The model under review builds one solid part; all positions refer to its coordinate system, in mm. A direction names the side the tool comes from. Give positions to 0.01 mm unless a question says otherwise; leave off trailing zeros. Order: outer loops, then holes, each group sorted by start corner. A loop starts at its lowest first (then second) coordinate and runs counter-clockwise, first axis right, second up. Notation, with made-up numbers: (-30, -15) - (-13, -15) arc R16 cw to (-13, 16) - close; hole circle Ø3 at (-36, 25). An arc over 180 degrees is marked (long way). Use CSV: the item, a comma, the result in double quotes.
```python
from build123d import *

# Parameters (mm, degrees)
PAD_DEPTH       = 1
PAD001_DEPTH    = 18
SKETCH002_W     = 19.2
SKETCH002_H     = 12.2
POCKET_DEPTH    = 5
SKETCH003_W     = 21.2
SKETCH003_H     = 14.2
SKETCH003_W_2   = 19.2
SKETCH003_H_2   = 12.2
PAD002_DEPTH    = 1
CHAMFER_SIZE    = 0.99
PAD003_DEPTH    = 2
CHAMFER001_SIZE = 1.8
SKETCH005_W     = 36
SKETCH005_H     = 15
PAD004_DEPTH    = 2.5
PAD004_FACE29_W = 15
PAD004_FACE29_H = 36
PAD005_DEPTH    = 10
SKETCH006_R     = 1
SKETCH006_R_2   = 0.751416
SKETCH006_R_3   = 0.769216
PAD006_DEPTH    = 1
SKETCH007_R     = 1.25
PAD007_DEPTH    = 1.2
PAD007_FACE39_W = 15
PAD007_FACE39_H = 36
POCKET001_DEPTH = 5
SKETCH008_R     = 6.15
POCKET002_DEPTH = 19
PAD008_DEPTH    = 1
PAD009_DEPTH    = 1
SKETCH009_W     = 12
SKETCH009_H     = 5
POCKET003_DEPTH = 5
FILLET_R        = 1
POCKET004_DEPTH = 5
POCKET005_DEPTH = 5


with BuildPart() as part:
    # Sketch → Pad (new body)
    with BuildSketch(Plane.XY):
        with BuildLine():
            Line((1, 0), (39, 0))
            ThreePointArc((39, 0), (39.707107, 0.292893), (40, 1))
            Line((40, 1), (40, 39))
            ThreePointArc((40, 39), (39.707107, 39.707107), (39, 40))
            Line((39, 40), (1, 40))
            ThreePointArc((1, 40), (0.292893, 39.707107), (0, 39))
            Line((0, 39), (0, 1))
            ThreePointArc((0, 1), (0.292893, 0.292893), (1, 0))
        make_face()
    extrude(amount=PAD_DEPTH)

    # Sketch001 (on Face10 of Pad) → Pad001 (join)
    with BuildSketch(Plane.XY.offset(1)):
        with BuildLine():
            Line((1, 0), (39, 0))
            ThreePointArc((39, 0), (39.707107, 0.292893), (40, 1))
            Line((40, 1), (40, 39))
            ThreePointArc((40, 39), (39.707107, 39.707107), (39, 40))
            Line((39, 40), (1, 40))
            ThreePointArc((1, 40), (0.292893, 39.707107), (0, 39))
            Line((0, 39), (0, 1))
            ThreePointArc((0, 1), (0.292893, 0.292893), (1, 0))
        make_face()
        with BuildLine():
            Line((2, 1), (38, 1))
            ThreePointArc((38, 1), (38.707107, 1.292893), (39, 2))
            Line((39, 2), (39, 38))
            ThreePointArc((39, 38), (38.707107, 38.707107), (38, 39))
            Line((38, 39), (2, 39))
            ThreePointArc((2, 39), (1.292893, 38.707107), (1, 38))
            Line((1, 38), (1, 2))
            ThreePointArc((1, 2), (1.292893, 1.292893), (2, 1))
        make_face(mode=Mode.SUBTRACT)
    extrude(amount=PAD001_DEPTH)

    # Sketch002 (on Face14 of Pad001) → Pocket (cut)
    with BuildSketch(Plane.YZ.offset(40)):
        with Locations((26.6, 11.1)):
            Rectangle(SKETCH002_W, SKETCH002_H)
    extrude(amount=-POCKET_DEPTH, mode=Mode.SUBTRACT)

    # Sketch003 (on Face17 of Pocket) → Pad002 (join)
    with BuildSketch(Plane(origin=(39, 0, 0), x_dir=(0, -1, 0), z_dir=(-1, 0, 0))):
        with Locations((-26.6, 11.1)):
            Rectangle(SKETCH003_W, SKETCH003_H)
        with Locations((-26.6, 11.1)):
            Rectangle(SKETCH003_W_2, SKETCH003_H_2, mode=Mode.SUBTRACT)
    extrude(amount=PAD002_DEPTH)

    # Chamfer
    chamfer_edges = [part.edges().sort_by_distance(p)[0] for p in [
        (38, 26.6, 18.2),
        (38, 16, 11.1),
        (38, 26.6, 4),
        (38, 37.2, 11.1),
    ]]
    chamfer(chamfer_edges, length=CHAMFER_SIZE)

    # Sketch004 (on Face11 of Chamfer) → Pad003 (join)
    with BuildSketch(Plane.XY.offset(1)):
        with BuildLine():
            Line((2, 39), (2, 18.5))
            ThreePointArc((2, 18.5), (2.292893, 17.792893), (3, 17.5))
            Line((3, 17.5), (5, 17.5))
            Line((5, 17.5), (5, 14))
            Line((5, 14), (17, 14))
            Line((17, 17.5), (17, 14))
            Line((17, 17.5), (19, 17.5))
            ThreePointArc((19, 17.5), (19.707107, 17.792893), (20, 18.5))
            Line((20, 18.5), (20, 20))
            Line((20, 20), (22, 20))
            Line((22, 20), (22, 17.5))
            Line((22, 17.5), (38, 17.5))
            Line((38, 17.5), (38, 38))
            Line((38, 38), (22, 38))
            Line((22, 38), (22, 37))
            Line((22, 37), (20, 37))
            Line((20, 37), (20, 39))
            Line((20, 39), (39, 39))
            Line((39, 1), (39, 39))
            Line((1, 1), (39, 1))
            Line((1, 39), (1, 1))
            Line((1, 39), (2, 39))
        make_face()
    extrude(amount=PAD003_DEPTH)

    # Chamfer001
    chamfer001_edges = [part.edges().sort_by_distance(p)[0] for p in [
        (11, 14, 3),
    ]]
    chamfer(chamfer001_edges, length=CHAMFER001_SIZE)

    # Sketch005 (on Face1 of Chamfer001) → Pad004 (join, symmetric)
    with BuildSketch(Plane.XY.offset(3)):
        with Locations((20, 8.5)):
            Rectangle(SKETCH005_W, SKETCH005_H)
    extrude(amount=PAD004_DEPTH, both=True)

    # Pad004 Face29 → Pad005 (add)
    with BuildSketch(Plane(origin=(20, 8.5, 5.5), x_dir=(0, 1, 0), z_dir=(0, 0, 1))):
        Rectangle(PAD004_FACE29_W, PAD004_FACE29_H)
    extrude(amount=PAD005_DEPTH)

    # Sketch006 (on Face18 of Pad005) → Pad006 (join)
    with BuildSketch(Plane.XY.offset(1)):
        with Locations((3, 18.5)):
            Circle(SKETCH006_R)
        with Locations((19, 18.5)):
            Circle(SKETCH006_R)
        with Locations((2.699211, 38.373474)):
            Circle(SKETCH006_R_2)
        with Locations((19.24682, 38.345665)):
            Circle(SKETCH006_R_3)
    extrude(amount=PAD006_DEPTH)

    # Sketch007 (on Face20 of Pad006) → Pad007 (join)
    with BuildSketch(Plane.XY.offset(1)):
        with Locations((35.5, 35.5)):
            Circle(SKETCH007_R)
        with Locations((35.5, 20)):
            Circle(SKETCH007_R)
    extrude(amount=PAD007_DEPTH)

    # Pad007 Face39 → Pocket001 (cut)
    with BuildSketch(Plane(origin=(20, 8.5, 15.5), x_dir=(0, 1, 0), z_dir=(0, 0, 1))):
        Rectangle(PAD007_FACE39_W, PAD007_FACE39_H)
    extrude(amount=-POCKET001_DEPTH, mode=Mode.SUBTRACT)

    # Sketch008 (on DatumPlane) → Pocket002 (cut, symmetric)
    with BuildSketch(Plane.YZ.offset(20)):
        with Locations((9, 11)):
            Circle(SKETCH008_R)
    extrude(amount=POCKET002_DEPTH, both=True, mode=Mode.SUBTRACT)

    # Pocket002 Face46 → Pad008 (add)
    with BuildSketch(Plane(origin=(2, 8.050341, 5.520041), x_dir=(0, 1, 0), z_dir=(-1, 0, 0))):
        with BuildLine():
            Line((7.949659, 2.520041), (-7.050341, 2.520041))
            Line((-7.050341, 2.520041), (-7.050341, -4.979959))
            Line((-7.050341, -4.979959), (-5.179982, -4.979959))
            ThreePointArc((-5.179982, -4.979959), (0.949659, 0.670041), (7.0793, -4.979959))
            Line((7.0793, -4.979959), (7.949659, -4.979959))
            Line((7.949659, -4.979959), (7.949659, 2.520041))
        make_face()
    extrude(amount=PAD008_DEPTH)

    # Pad008 Face32 → Pad009 (add)
    with BuildSketch(Plane(origin=(38, 8.050341, 5.520041), x_dir=(0, -1, 0), z_dir=(1, 0, 0))):
        with BuildLine():
            Line((7.050341, 2.520041), (-7.949659, 2.520041))
            Line((-7.949659, 2.520041), (-7.949659, -4.979959))
            Line((-7.949659, -4.979959), (-7.0793, -4.979959))
            ThreePointArc((-7.0793, -4.979959), (-0.949659, 0.670041), (5.179982, -4.979959))
            Line((5.179982, -4.979959), (7.050341, -4.979959))
            Line((7.050341, -4.979959), (7.050341, 2.520041))
        make_face()
    extrude(amount=PAD009_DEPTH)

    # Sketch009 (on Face69 of Pad009) → Pocket003 (cut)
    with BuildSketch(Plane.XY.offset(10.5)):
        with Locations((11, 13.5)):
            Rectangle(SKETCH009_W, SKETCH009_H)
    extrude(amount=-POCKET003_DEPTH, mode=Mode.SUBTRACT)

    # Fillet
    fillet_edges = [part.edges().sort_by_distance(p)[0] for p in [
        (11, 16, 5.5),
    ]]
    fillet(fillet_edges, radius=FILLET_R)

    # Sketch010 (on Face62 of Fillet) → Pocket004 (cut)
    with BuildSketch(Plane(origin=(0, 0, 0), x_dir=(0, -1, 0), z_dir=(-1, 0, 0))):
        with BuildLine():
            ThreePointArc((-22.577213, 15.673276), (-21.827213, 14.923276), (-21.077213, 15.673276))
            Line((-21.077213, 15.673276), (-21.077213, 20.673276))
            ThreePointArc((-21.077213, 20.673276), (-21.827213, 21.423276), (-22.577213, 20.673276))
            Line((-22.577213, 15.673276), (-22.577213, 20.673276))
        make_face()
    extrude(amount=-POCKET004_DEPTH, mode=Mode.SUBTRACT)

    # Sketch013 (on Face63 of Pocket004) → Pocket005 (cut)
    with BuildSketch(Plane(origin=(0, 40, 0), x_dir=(-1, 0, 0), z_dir=(0, 1, 0))):
        with BuildLine():
            Line((-6.1, 4), (-6.1, 6))
            ThreePointArc((-6.1, 6), (-6.392893, 6.707107), (-7.1, 7))
            Line((-7.1, 7), (-15.1, 7))
            ThreePointArc((-15.1, 7), (-15.807107, 6.707107), (-16.1, 6))
            Line((-16.1, 6), (-16.1, 4))
            ThreePointArc((-16.1, 4), (-15.807107, 3.292893), (-15.1, 3))
            Line((-15.1, 3), (-7.1, 3))
            ThreePointArc((-7.1, 3), (-6.392893, 3.292893), (-6.1, 4))
        make_face()
    extrude(amount=-POCKET005_DEPTH, mode=Mode.SUBTRACT)


solid = part.part
```
Item 1: Tool access review of faces 4 (the face through (0.5, 22.577, 17.3)), 5 (the face through (39, 17, 11)), 6 (the face through (3, 38, 2)): name each direction out of +Z, -Z, +X, -X, +Y, -Y from which nothing blocks a thin tool from reaching the whole face with its end or side.
Results list:
face 4,"+Z, -X"
face 5,"+X"
face 6,"+Z"
Item 2: Take a section at B-B, the plane x = 13. Give the boundary of the cut face in (y, z), and give its area (3 significant figures).
Results list:
outline,"(0, 0) - (40, 0) - (40, 3) - (39, 3) - (39, 1) - (16, 1) - (16, 4.5) arc R1 ccw to (15, 5.5) - (11.75, 5.5) arc R6.15 cw to (2.87, 10.5) - (1, 10.5) - (1, 19) - (0, 19) - close; (39, 7) - (40, 7) - (40, 19) - (39, 19) - close"
area,"151 mm2"
Item 3: Clearance check with flat-ended pins moving along their axes: pin 1 (11.5 mm diameter, centred on x = 18, y = 29.5, fed in from +Z); pin 2 (4.5 mm diameter, centred on x = 3.5, y = 27.5, fed in from +Z); pin 3 (1 mm diameter, centred on x = 10, y = 13.5, fed in from +Z). State where each tip first meets the part, or that it passes through.
Results list:
pin 1,"stops at z = 1"
pin 2,"stops at z = 3"
pin 3,"stops at z = 5.5"
Item 4: Take a section at C-C, the plane x = 35.5. Give the boundary of the cut face in (y, z).
Results list:
outline,"(0, 0) - (40, 0) - (40, 19) - (39, 19) - (39, 3) - (38, 3) - (38, 1) - (36.75, 1) - (36.75, 2.2) - (34.25, 2.2) - (34.25, 1) - (21.25, 1) - (21.25, 2.2) - (18.75, 2.2) - (18.75, 1) - (17.5, 1) - (17.5, 3) - (16, 3) - (16, 10.5) - (15.13, 10.5) arc R6.15 cw to (2.87, 10.5) - (1, 10.5) - (1, 19) - (0, 19) - close"
Item 5: Wall thickness on L1, parallel to X at y = 9.5, z = 11.5; L2, parallel to Y at x = 26, z = 4.75: over which ranges is each line inside the solid? List them lowest first.
Results list:
L1,"x = 0 to 1, 39 to 40"
L2,"y = 0 to 16, 39 to 40"
Item 6: Mouldability with a two-part tool opening along X and no side actions: class faces 1 (the face through (39.715, 39.699, 9.367)), 2 (the face through (20, 28, 1)), 3 (the face through (20, 20, 0)) as pulls with the +X half, pulls with the -X half, needs draft (parallel to the pull), parting line crosses it, or undercut.
Results list:
face 1,"pulls with the +X half"
face 2,"undercut"
face 3,"needs draft"
